The model under review builds one solid part; all positions refer to its coordinate system, in mm. Face numbers are marked on the shaded views. A direction names the side the tool comes from. Round coordinates to 2 decimals unless told otherwise and drop trailing zeros. Order: outer loops, then holes, each group sorted by start corner. A loop starts at its lowest first (then second) coordinate and runs counter-clockwise, first axis right, second up.
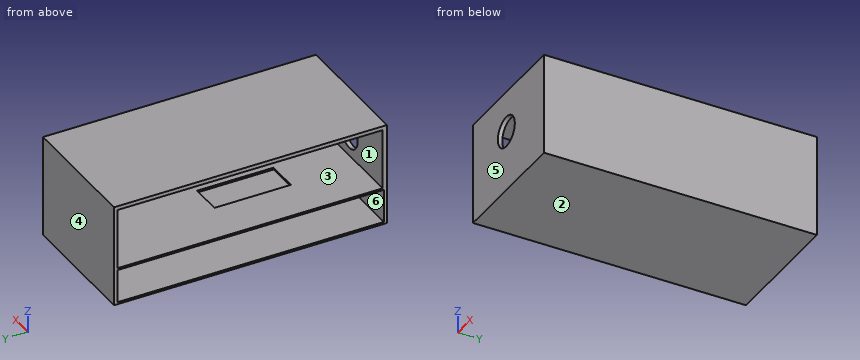
from build123d import *

# Parameters (mm, degrees)
F0_W           = 101.6
F0_H           = 203.2
F1_DEPTH       = 76.2
F2_W           = 96.435938
F2_H           = 70.576824
F3_DEPTH       = 258.572
F4_W           = 101.6
F4_H           = 76.2
F5_DEPTH       = 3.302
F6_R           = 11.433627
F7_DEPTH       = 25.4
F8_W           = 100.535084
F8_H           = 27.989352
F9_DEPTH       = 203.2
F10_W          = 96.052602
F10_H          = 24.980713
F11_DEPTH      = 200.914
F12_W          = 23.410334
F12_H          = 56.895998
F13_DEPTH      = 9.652
F13_DEPTH_BACK = 11.938
F14_W          = 233.204983
F14_H          = 100.407705
F15_DEPTH      = 5.842
F16_W          = 95.758
F16_H          = 76.2
F17_DEPTH      = 2.794


with BuildPart() as f1:
    # F0 (on Top) → F1 (new body)
    with BuildSketch(Plane.XY):
        Rectangle(F0_W, F0_H)
    extrude(amount=F1_DEPTH)

    # F2 (on face) → F3 (cut)
    with BuildSketch(Plane.XZ.offset(101.6)):
        with Locations((0.141935, 37.975889)):
            Rectangle(F2_W, F2_H)
    extrude(amount=-F3_DEPTH, mode=Mode.SUBTRACT)

    # F4 (on face) → F5 (join)
    with BuildSketch(Plane.XZ.offset(101.6)):
        with Locations((0, 38.1)):
            Rectangle(F4_W, F4_H)
    extrude(amount=-F5_DEPTH)

    # F6 (on face) → F7 (cut)
    with BuildSketch(Plane.XZ.offset(101.6)):
        with Locations((0, 45.440793)):
            Circle(F6_R)
    extrude(amount=-F7_DEPTH, mode=Mode.SUBTRACT)

    # F8 (on face) → F9 (join)
    with BuildSketch(Plane(origin=(0, 101.6, 0), x_dir=(-1, 0, 0), z_dir=(0, 1, 0))):
        with Locations((-0.532458, 13.994676)):
            Rectangle(F8_W, F8_H)
    extrude(amount=-F9_DEPTH)

    # F10 (on face) → F11 (cut)
    with BuildSketch(Plane(origin=(0, 101.6, 0), x_dir=(-1, 0, 0), z_dir=(0, 1, 0))):
        with Locations((-0.199899, 14.034254)):
            Rectangle(F10_W, F10_H)
    extrude(amount=-F11_DEPTH, mode=Mode.SUBTRACT)

    # F12 (on face) → F13 (cut, two sides)
    with BuildSketch(Plane.XY.offset(27.989352)) as f13_sk:
        with Locations((-0.740831, -19.557999)):
            Rectangle(F12_W, F12_H)
    extrude(amount=-F13_DEPTH, mode=Mode.SUBTRACT)
    extrude(f13_sk.sketch, amount=-F13_DEPTH_BACK, mode=Mode.SUBTRACT)

    # F14 (on face) → F15 (cut)
    with BuildSketch(Plane(origin=(-50.8, 0, 0), x_dir=(0, -1, 0), z_dir=(-1, 0, 0))):
        with Locations((6.751563, 32.170609)):
            Rectangle(F14_W, F14_H)
    extrude(amount=-F15_DEPTH, mode=Mode.SUBTRACT)

    # F16 (on face) → F17 (join)
    with BuildSketch(Plane(origin=(0, 101.6, 0), x_dir=(-1, 0, 0), z_dir=(0, 1, 0))):
        with Locations((-2.921, 38.1)):
            Rectangle(F16_W, F16_H)
    extrude(amount=-F17_DEPTH)


solid = f1.part
(1) We need section D-D (x = 0). Give the boundary of the cut face in (y, z), and give its area (3 significant figures).
(2) We need section B-B (x = 27). Give the boundary of the cut face in (y, z), and give its area (3 significant figures).
(3) We need section A-A (y = -16). Give the boundary of the cut face in (x, z).
(4) Clearance check with flat-ended pins moving along their axes: P1, Ø13.5, axis at y = -33.5, z = 40, coming from the -X side; P2, Ø13.5, axis at x = 0, z = 45.44, coming from the -Y side; P3, Ø20, axis at y = 17, z = 15, coming from the -X side. State where each tip first meets the part, or that it passes through.
(5) We need section C-C (z = 39.5). Give the boundary of the cut face in (x, y), and give its area (3 significant figures).
(6) To check wall thickness, follow L1, parallel to Z at x = 34, y = -54.5; L2, parallel to Y at x = 8, z = 5; L3, parallel to Y at x = -25, z = 37. State the ranges of each line that lie inside material, in increasing order.
(7) Tool access review of the marked faces 5 and 6: name each direction out of +Z, -Z, +X, -X, +Y, -Y from which nothing blocks a thin tool from reaching the whole face with its end or side.
(8) The part is to be moulded in two halves that separate along Z. For the marked faces 1, 2, 3 and 4, say which applies: pulls with the +Z half, pulls with the -Z half, needs draft (parallel to the pull), parting line crosses it, or undercut.
Verdict:
1. outline: (-101.6, 0) - (101.6, 0) - (101.6, 76.2) - (-101.6, 76.2) - (-101.6, 56.87) - (-98.3, 56.87) - (-98.3, 73.26) - (98.81, 73.26) - (98.81, 27.99) - (8.89, 27.99) - (8.89, 26.52) - (98.81, 26.52) - (98.81, 1.54) - (-99.31, 1.54) - (-99.31, 26.52) - (-48.01, 26.52) - (-48.01, 27.99) - (-98.3, 27.99) - (-98.3, 34.01) - (-101.6, 34.01) - close
1. area: 1,450 mm2
2. outline: (-101.6, 0) - (101.6, 0) - (101.6, 76.2) - (-101.6, 76.2) - close; hole (-99.31, 1.54) - (98.81, 1.54) - (98.81, 26.52) - (-99.31, 26.52) - close; hole (-98.3, 27.99) - (98.81, 27.99) - (98.81, 73.26) - (-98.3, 73.26) - close
2. area: 1,610 mm2
3. outline: (-44.96, 0) - (50.8, 0) - (50.8, 76.2) - (-44.96, 76.2) - (-44.96, 73.26) - (48.36, 73.26) - (48.36, 27.99) - (10.96, 27.99) - (10.96, 26.52) - (48.23, 26.52) - (48.23, 1.54) - (-44.96, 1.54) - close; (-44.96, 26.52) - (-12.45, 26.52) - (-12.45, 27.99) - (-44.96, 27.99) - close
4. P1: stops at x = 48.36
4. P2: stops at y = 98.81
4. P3: stops at x = 48.23
5. outline: (-44.96, -101.6) - (-9.77, -101.6) - (-9.77, -98.3) - (-44.96, -98.3) - close; (-44.96, 98.81) - (48.36, 98.81) - (48.36, -98.3) - (9.77, -98.3) - (9.77, -101.6) - (50.8, -101.6) - (50.8, 101.6) - (-44.96, 101.6) - close
5. area: 1,000 mm2
6. L1: z = 0 to 1.54, 26.52 to 27.99, 73.26 to 76.2
6. L2: y = -101.6 to -99.31, 98.81 to 101.6
6. L3: y = -101.6 to -98.3, 98.81 to 101.6
7. face 5: +Z, -Z, +X, -X, -Y
7. face 6: -X
8. face 1: undercut
8. face 2: pulls with the -Z half
8. face 3: undercut
8. face 4: needs draft
